Design review of the part built by this model. Coordinates are the model's own, in mm. A direction names the side the tool comes from. Coordinates: 2 decimals unless noted, no trailing zeros. Loops run counter-clockwise (first coordinate to the right, second up) from the corner with the lowest first, then second, coordinate; pieces in that order, holes last. Notation, with made-up numbers: M -13,87.25 L -6,87.25 A18 cw -6,95.25 Z; hole C 24,69 d11. An arc over 180 degrees is marked long. Answer as a JSON object with one key per item and string values. Group by question number.
1. Insertion check: pin 1 (8 mm diameter, centred on x = -39, z = 5, fed in from +Y); pin 2 (8 mm diameter, centred on x = 81, z = 13, fed in from -Y); pin 3 (1.5 mm diameter, centred on x = 61, z = 22, fed in from +Y); pin 4 (4 mm diameter, centred on x = -49.8, y = 65.8, fed in from -Z). Each pin has a flat end and moves straight along its axis. Give the tip position at first contact, or say it passes through.
2. Consider section C-C (x = -10.5). State the section outline as (y, z) points, then the cut area to 3 significant figures.
3. Consider section B-B (x = 39.5). State the section outline as (y, z) points.
4. Consider section D-D (y = 88). State the section outline as (x, z) points, then the cut area to 3 significant figures.
5. Draft analysis for pull direction Y (two halves, no side actions). For faces 5 (the cylindrical face through (-53, 26.76, 1.23)), 6 (the cylindrical face through (-49.21, 94.22, 16.03)), 7 (the flat face through (-21, -50, 2)), state which applies: +Y half, -Y half, draft (parallel to the pull), parting line (faces both ways), or undercut.
6. To check wall thickness, follow probe 1 along X at (y, z) = (65.8, 5.5); probe 2 along X at (y, z) = (59, 28); probe 3 along X at (y, z) = (-25, 37.5). State the ranges of each line that lie inside material, in increasing order.
7. Machinability: for faces 1 (the flat face through (-7, 98, 40)), 2 (the flat face through (-80, 0, 20)), 3 (the flat face through (-87.5, 43, 21)), 4 (the flat face through (-67.5, -28, 21)), which of the approach directions +Z, -Z, +X, -X, +Y, -Y give a long, thin tool a straight path to every point of the face, cutting with its end or side? Answer none if there is none.
8. Consider section A-A (y = 37). State the section outline as (x, z) points, then the cut area to 4 significant figures.
from build123d import *

# Parameters (mm, degrees)
F1_DEPTH  = 40
F2_W      = 100
F2_H      = 200
F3_DEPTH  = 100
F4_R      = 5
F5_T      = -2.5
F6_R      = 6
F7_DEPTH  = 25
F8_R      = 3
F9_DEPTH  = 25
F10_R     = 8
F11_DEPTH = 25
F12_R     = 5
F13_DEPTH = 25
F14_R     = 3
F14_R_2   = 1.25
F15_DEPTH = 10
F16_R     = 3
F17_DEPTH = 150
F18_W     = 15
F18_H     = 6
F19_DEPTH = 250
F20_R     = 1.5
F21_DEPTH = 12.5


with BuildPart() as f1:
    # F0 (on Top) → F1 (new body)
    with BuildSketch(Plane.XY):
        with BuildLine():
            Line((-90, 83.2380757938), (-90, -50))
            Line((-90, -50), (90, -50))
            Line((90, -50), (90, 83.2380757938))
            ThreePointArc((90, 83.2380757938), (45.7737973711, 95.7737973711), (0, 100))
            ThreePointArc((0, 100), (-45.7737973711, 95.7737973711), (-90, 83.2380757938))
        make_face()
    extrude(amount=F1_DEPTH)

    # F2 (on Top) → F3 (cut)
    with BuildSketch(Plane.XY):
        with Locations((-120, -100)):
            Rectangle(F2_W, F2_H)
        with Locations((120, -100)):
            Rectangle(F2_W, F2_H)
    extrude(amount=F3_DEPTH, mode=Mode.SUBTRACT)

    # F4
    f4_edges = [f1.edges().sort_by_distance(p)[0] for p in [
        (-90, 83.238076, 20),
        (90, 83.238076, 20),
        (90, 0, 20),
        (70, 0, 20),
        (-90, 0, 20),
        (-70, 0, 20),
    ]]
    fillet(f4_edges, radius=F4_R)

    # F5
    f5_openings = [f1.faces().sort_by_distance(p)[0] for p in [
        (0, 26.262097, 40),
        (0, -50, 20),
    ]]
    offset(amount=F5_T, openings=f5_openings)

    # F6 (on Top) → F7 (cut)
    with BuildSketch(Plane.XY):
        with Locations((0, -30)):
            Circle(F6_R)
    extrude(amount=F7_DEPTH, mode=Mode.SUBTRACT)

    # F8 (on Top) → F9 (cut)
    with BuildSketch(Plane.XY):
        with Locations((-55.8614357137, 25.8614357137)):
            Circle(F8_R)
        with Locations((55.8614357137, 25.8614357137)):
            Circle(F8_R)
    extrude(amount=F9_DEPTH, mode=Mode.SUBTRACT)

    # F10 (on Top) → F11 (join)
    with BuildSketch(Plane.XY):
        with Locations((-81, 77)):
            Circle(F10_R)
        with Locations((81, 77)):
            Circle(F10_R)
    extrude(amount=F11_DEPTH)

    # F12 (on Top) → F13 (cut)
    with BuildSketch(Plane.XY):
        with Locations((-81, 77)):
            Circle(F12_R)
        with Locations((81, 77)):
            Circle(F12_R)
    extrude(amount=F13_DEPTH, mode=Mode.SUBTRACT)

    # F14 (on Top) → F15 (join)
    with BuildSketch(Plane.XY):
        with Locations((-65, 15)):
            Circle(F14_R)
        with Locations((-65, 15)):
            Circle(F14_R_2, mode=Mode.SUBTRACT)
        with Locations((-49.8, 65.8)):
            Circle(F14_R)
        with Locations((-49.8, 65.8)):
            Circle(F14_R_2, mode=Mode.SUBTRACT)
        with Locations((-21.9, 65.8)):
            Circle(F14_R)
        with Locations((-21.9, 65.8)):
            Circle(F14_R_2, mode=Mode.SUBTRACT)
        with Locations((-16.8, 13.7)):
            Circle(F14_R)
        with Locations((-16.8, 13.7)):
            Circle(F14_R_2, mode=Mode.SUBTRACT)
    extrude(amount=F15_DEPTH)

    # F16 (on Front) → F17 (cut, symmetric)
    with BuildSketch(Plane.XZ):
        with Locations((47, 14)):
            Circle(F16_R)
        with Locations((-47, 14)):
            Circle(F16_R)
    extrude(amount=F17_DEPTH, both=True, mode=Mode.SUBTRACT)

    # F18 (on Front) → F19 (cut)
    with BuildSketch(Plane.XZ):
        with Locations((0, 5.5)):
            Rectangle(F18_W, F18_H)
    extrude(amount=-F19_DEPTH, mode=Mode.SUBTRACT)

    # F20 (on Top) → F21 (cut, symmetric)
    with BuildSketch(Plane.XY):
        with Locations((-3, 95)):
            Circle(F20_R)
        with Locations((3, 95)):
            Circle(F20_R)
    extrude(amount=F21_DEPTH, both=True, mode=Mode.SUBTRACT)


solid = f1.part
Findings below:
{
 "1": {"pin 1": "stops at y = 97.54", "pin 2": "stops at y = 0", "pin 3": "stops at y = 92.63", "pin 4": "stops at z = 0"},
 "2": {"outline": "M -50,0 L 99.78,0 L 99.78,40 L 97.28,40 L 97.28,2.5 L -50,2.5 Z", "area": "468 mm^2"},
 "3": {"outline": "M -50,0 L 96.86,0 L 96.86,40 L 94.33,40 L 94.33,2.5 L -50,2.5 Z"},
 "4": {"outline": "M -76.52,0 L 76.52,0 L 76.52,40 L 67.91,40 L 67.91,2.5 L -67.91,2.5 L -67.91,40 L -76.52,40 Z", "area": "1,030 mm^2"},
 "5": {"face 5": "undercut", "face 6": "draft", "face 7": "-Y half"},
 "6": {"probe 1": "x = -90 to -87.5, -52.8 to -51.05, -48.55 to -46.8, -24.9 to -23.15, -20.65 to -18.9, 87.5 to 90", "probe 2": "x = -90 to -87.5, 87.5 to 90", "probe 3": "x = -70 to -67.5, 67.5 to 70"},
 "7": {"face 1": "+Z, +X, -X, +Y, -Y", "face 2": "+Z, -Z, -X, -Y", "face 3": "+Z", "face 4": "+Z, -Y"},
 "8": {"outline": "M -90,0 L 90,0 L 90,40 L 87.5,40 L 87.5,2.5 L -87.5,2.5 L -87.5,40 L -90,40 Z", "area": "637.5 mm^2"}
}
